Input: part model. Units: mm. Frame: model coordinates. A direction names the side the tool comes from. Give positions to 0.01 mm unless a question says otherwise; leave off trailing zeros. Loops run counter-clockwise (first coordinate to the right, second up) from the corner with the lowest first, then second, coordinate; pieces in that order, holes last.
Autodesk Inventor part; units mm, degrees
ref_plane "YZ Plane" through (0, 0, 0) normal (1, 0, 0) x (0, 1, 0)
ref_plane "XZ Plane" through (0, 0, 0) normal (0, 1, 0) x (-1, 0, 0)
ref_plane "XY Plane" through (0, 0, 0) normal (0, 0, 1) x (1, 0, 0)
sketch "Sketch1" plane through (0, 0, 0) normal (0, 1, 0) x (-1, 0, 0)
  line L0 (0, 0) -> (-22.86, 0)
  line L1 (-22.86, 0) -> (-22.86, -22.86)
  line L2 (-22.86, -22.86) -> (0, -22.86)
  line L3 (0, -22.86) -> (0, 0)
  line L4 (-22.86, -22.86) -> (-19.304, -22.86)
  line L5 (-19.304, -22.86) -> (-19.304, -19.304) construction
  line L6 (-19.304, -19.304) -> (-22.86, -19.304) construction
  line L7 (-22.86, -19.304) -> (-22.86, -22.86)
  line L8 (0, -22.86) -> (-3.556, -22.86)
  line L9 (-3.556, -22.86) -> (-3.556, -19.304) construction
  line L10 (-3.556, -19.304) -> (0, -19.304) construction
  line L11 (0, -19.304) -> (0, -22.86)
  line L12 (0, 0) -> (-3.556, 0)
  line L13 (-3.556, 0) -> (-3.556, -3.556) construction
  line L14 (-3.556, -3.556) -> (0, -3.556) construction
  line L15 (0, -3.556) -> (0, 0)
  line L16 (-22.86, 0) -> (-19.304, 0)
  line L17 (-19.304, 0) -> (-19.304, -3.556) construction
  line L18 (-19.304, -3.556) -> (-22.86, -3.556) construction
  line L19 (-22.86, -3.556) -> (-22.86, 0)
  circle A0 centre (-3.556, -19.304) radius 2.032
  circle A1 centre (-19.304, -19.304) radius 2.032
  circle A2 centre (-19.304, -3.556) radius 2.032
  circle A3 centre (-3.556, -3.556) radius 2.032
  line L20 (-3.556, -19.304) -> (-19.304, -19.304)
  line L21 (-19.304, -19.304) -> (-19.304, -3.556)
  line L22 (-19.304, -3.556) -> (-3.556, -3.556)
  line L23 (-3.556, -3.556) -> (-3.556, -19.304)
  dimension "d0" = 22.86
  dimension "d1" = 22.86
  dimension "d2" = 3.556
  dimension "d3" = 3.556
  dimension "d4" = 3.556
  dimension "d5" = 3.556
  dimension "d6" = 3.556
  dimension "d7" = 3.556
  dimension "d8" = 3.556
  dimension "d9" = 3.556
  dimension "d10" = 4.064
  dimension "d11" = 4.064
  dimension "d12" = 4.064
  dimension "d13" = 4.064
extrude "Extrusion1" add sketch "Sketch1" along normal blind 2.032 contours L3 L2 L1 L0 | A0 L20 A1 L21 A2 L22 A3 L23
fillet "Fillet1" radius 2 4 edges at (0, 1.016, 0) (22.86, 1.016, 0) (22.86, 1.016, -22.86) (0, 1.016, -22.86)
sketch "Sketch2" plane through (0, 2.032, 0) normal (0, 1, 0) x (1, 0, 0)
  line L0 (9.398, 13.843) -> (13.462, 13.843)
  line L1 (13.462, 13.843) -> (13.462, 9.017)
  line L2 (13.462, 9.017) -> (9.398, 9.017)
  line L3 (9.398, 9.017) -> (9.398, 13.843)
  line L4 (9.398, 13.843) -> (13.462, 9.017) construction
  line L5 (13.462, 13.843) -> (9.398, 9.017) construction
  line L6 (22.86, 2) -> (22.86, 20.86)
  line L7 (20.86, 22.86) -> (2, 22.86)
  point P0 (0, 0)
  point P1 (11.43, 11.43)
  dimension "d17" = 4.064
  dimension "d18" = 4.826
  dimension "d19" = 11.43
  dimension "d20" = 11.43
extrude "Extrusion2" add sketch "Sketch2" along normal blind 1.016
properties part number "as5600"
(1) Reachability of faces 5 (the flat face through (9.398, 2.5, -11.4)), 6 (the cylindrical face through (0.57, 1.03, -0.6)), 7 (the flat face through (11.4, 2.5, -13.843)) from +Z, -Z, +X, -X, +Y, -Y: full face, straight path, thin tool, end or side. Return the list, or none.
Values follow:
face 5: +Z, -Z, -X, +Y
face 6: +Z, -X, +Y, -Y
face 7: -Z, +X, -X, +Y
(2) Pin query (flat end, axial travel): pin 1 Ø0.8 at (y, z) = (2.5, -11) entering from +X; pin 2 Ø8 at (x, z) = (4.5, -14) entering from +Y; pin 3 Ø0.8 at (x, y) = (11, 2.5) entering from +Z. Return the tip coordinate at first contact, or that it passes through.
Values follow:
pin 1: stops at x = 13.46
pin 2: stops at y = 2.03
pin 3: stops at z = -9.02
(3) Cut plane A-A (z = -13.25). Return the cut outline in (x, y), and give its area (3 significant figures).
Values follow:
outline: (0, 0) - (22.86, 0) - (22.86, 2.03) - (13.46, 2.03) - (13.46, 3.05) - (9.4, 3.05) - (9.4, 2.03) - (0, 2.03) - close
area: 50.6 mm2
(4) Ray query, probe 1 along Z at (x, y) = (3.5, 0.7); probe 2 along Z at (x, y) = (19.75, 0.95); probe 3 along X at (y, z) = (0.25, -5). Return the intervals inside material, ascending.
Values follow:
probe 1: z = -22.86 to -21.34, -17.27 to -5.59, -1.52 to 0
probe 2: z = -22.86 to -21.29, -17.32 to -5.54, -1.57 to 0
probe 3: x = 0 to 2.13, 4.99 to 17.87, 20.73 to 22.86
(5) Cut plane D-D (y = 0.55). Return the cut outline in (x, z).
Values follow:
outline: (0, -20.86) arc R2 ccw to (2, -22.86) - (20.86, -22.86) arc R2 ccw to (22.86, -20.86) - (22.86, -2) arc R2 ccw to (20.86, 0) - (2, 0) arc R2 ccw to (0, -2) - close; hole circle Ø4.06 at (3.56, -19.3); hole circle Ø4.06 at (3.56, -3.56); hole circle Ø4.06 at (19.3, -19.3); hole circle Ø4.06 at (19.3, -3.56)
(6) Cut plane C-C (z = -20.25). Return the cut outline in (x, y).
Values follow:
outline: (0, 0) - (1.76, 0) - (1.76, 2.03) - (0, 2.03) - close; (5.35, 0) - (17.51, 0) - (17.51, 2.03) - (5.35, 2.03) - close; (21.1, 0) - (22.86, 0) - (22.86, 2.03) - (21.1, 2.03) - close
(7) Mould query, pull axis Z, two halves, no side actions, for faces 1 (the cylindrical face through (5.17, 1, -2.32)), 2 (the cylindrical face through (0.6, 1.03, -22.29)), 3 (the flat face through (13.462, 2.5, -11.5)), 4 (the cylindrical face through (17.366, 1.002, -4.166)). Classes: +Z half, -Z half, draft (parallel to the pull), parting line (faces both ways), or undercut.
Values follow:
face 1: undercut
face 2: -Z half
face 3: draft
face 4: undercut
(8) Cut plane B-B (x = 4.5). Return the cut outline in (y, z), and give its area (3 significant figures).
Values follow:
outline: (0, -22.86) - (2.03, -22.86) - (2.03, -21.1) - (0, -21.1) - close; (0, -17.5) - (2.03, -17.5) - (2.03, -5.36) - (0, -5.36) - close; (0, -1.76) - (2.03, -1.76) - (2.03, 0) - (0, 0) - close
area: 31.8 mm2
